Verification items for the finished model (mm, model axes). Round coordinates to 2 decimals unless told otherwise and drop trailing zeros. Write each loop counter-clockwise with the first axis right and the second up, starting at its lowest first coordinate (ties: lowest second). Pieces come first, ordered by that corner, then holes. Notation, with made-up numbers: (35.5, 13.25) - (56.5, 13.25) arc R25 ccw to (56.5, 35.25) - close; hole circle Ø1 at (26.25, 3.5). An arc over 180 degrees is marked (long way). Write each question's results on one line, items separated by ' | '.
```python
from build123d import *

# Parameters (mm, degrees)
F0_R     = 38.1
F1_DEPTH = 25.4
F3_D     = 12.7
F4_R     = 6.35
F5_R     = 6.35


with BuildPart() as f1:
    # F0 (on Right) → F1 (new body)
    with BuildSketch(Plane.YZ):
        Circle(F0_R)
    extrude(amount=F1_DEPTH)

    # F3 (through all)
    with Locations(Plane.YZ.offset(25.4)):
        with Locations((0, 0)):
            Hole(F3_D / 2)

    # F4
    f4_edges = [f1.edges().sort_by_distance(p)[0] for p in [
        (25.4, -38.1, 0),
    ]]
    fillet(f4_edges, radius=F4_R)

    # F5
    f5_edges = [f1.edges().sort_by_distance(p)[0] for p in [
        (0, -38.1, 0),
    ]]
    fillet(f5_edges, radius=F5_R)


solid = f1.part
```
(1) Go/stop test with flat-tipped pins: pin 1 Ø6 at (x, z) = (21, -15.5) entering from -Y; pin 2 Ø12 at (x, z) = (18, 13.5) entering from +Y; pin 3 Ø3 at (x, z) = (17.5, -21) entering from -Y. Record where each tip stops, or that it passes through.
Answer:
pin 1: y = -35.86 | pin 2: y = 37.35 | pin 3: y = -32.73
(2) Section check A-A (z = 0). Record the cut outline in (x, y).
Answer:
outline: (0, -31.75) arc R6.35 ccw to (6.35, -38.1) - (19.05, -38.1) arc R6.35 ccw to (25.4, -31.75) - (25.4, -6.35) - (0, -6.35) - close; (0, 6.35) - (25.4, 6.35) - (25.4, 31.75) arc R6.35 ccw to (19.05, 38.1) - (6.35, 38.1) arc R6.35 ccw to (0, 31.75) - close
(3) Section check D-D (x = 21.25). Record the cut outline in (y, z), plus the area to 3 significant figures.
Answer:
outline: circle Ø75.41 at (0, 0); hole circle Ø12.7 at (0, 0) | area: 4,340 mm2
(4) Thickness scan on L1, parallel to Z at x = 16.75, y = 0; L2, parallel to X at y = 1, z = 32; L3, parallel to Z at x = 4.5, y = -15.5. Record the ranges inside material, lowest first.
Answer:
L1: -38.1 to -6.35, 6.35 to 38.1 | L2: 0.01 to 25.39 | L3: -34.5 to 34.5
(5) Mould release check, pull along Y, two halves, no side actions. Record for faces 1 (the cylindrical face through (12.611, -30.235, -23.183)), 2 (the cylindrical face through (12.52, 1.38, -6.2)), 3 (the flat face through (25.4, 0, -7)): released by +Y, released by -Y, zero draft, split by the parting line, or undercut.
Answer:
face 1: split by the parting line | face 2: undercut | face 3: zero draft
(6) Section check C-C (x = 10.75). Record the cut outline in (y, z), plus the area to 3 significant figures.
Answer:
outline: circle Ø76.2 at (0, 0); hole circle Ø12.7 at (0, 0) | area: 4,430 mm2
